```python
from build123d import *

# Parameters (mm, degrees)
F0_R     = 30
F1_DEPTH = 10
F2_R     = 2.5
F3_DEPTH = 10.001
F4_R     = 9
F5_DEPTH = 1.5
F6_R     = 7.5
F7_DEPTH = 10


with BuildPart() as f1:
    # F0 (on Top) → F1 (new body)
    with BuildSketch(Plane.XY):
        Circle(F0_R)
    extrude(amount=F1_DEPTH)

    # F2 (on face) → F3 (cut, through all)
    with BuildSketch(Plane.XY.offset(10)):
        with BuildLine():
            ThreePointArc((0, 23), (1.767767, 23.732233), (2.5, 25.5))
            ThreePointArc((2.5, 25.5), (-1.767767, 27.267767), (0, 23))
        make_face()
        with Locations((25.5, 0)):
            Circle(F2_R)
        with Locations((0, -25.5)):
            Circle(F2_R)
        with Locations((-25.5, 0)):
            Circle(F2_R)
    extrude(amount=-F3_DEPTH, mode=Mode.SUBTRACT)

    # F4 (on face) → F5 (join)
    with BuildSketch(Plane(origin=(0, 0, 0), x_dir=(1, 0, 0), z_dir=(0, 0, -1))):
        Circle(F4_R)
    extrude(amount=F5_DEPTH)

    # F6 (on face) → F7 (join)
    with BuildSketch(Plane(origin=(0, 0, -1.5), x_dir=(1, 0, 0), z_dir=(0, 0, -1))):
        Circle(F6_R)
    extrude(amount=F7_DEPTH)


solid = f1.part
```
Build history of the part. All positions in model axes, mm. A direction names the side the tool comes from. Round coordinates to 2 decimals unless told otherwise and drop trailing zeros. Order: outer loops, then holes, each group sorted by start corner. A loop starts at its lowest first (then second) coordinate and runs counter-clockwise, first axis right, second up. Notation, with made-up numbers: (36.5, 1) -> (51.5, 1) arc R24 cw to (51.5, 21) -> close; hole circle Ø3 at (-2, 5.25). An arc over 180 degrees is marked (long way). Answer in a Markdown table with one row per item.
1) Band-saw the part on A-A on y = 0. Give the cut face in (x, z).
Values:
| item | result |
|---|---|
| outline | (-30, 0) -> (-28, 0) -> (-28, 10) -> (-30, 10) -> close; (-23, 0) -> (-9, 0) -> (-9, -1.5) -> (-7.5, -1.5) -> (-7.5, -11.5) -> (7.5, -11.5) -> (7.5, -1.5) -> (9, -1.5) -> (9, 0) -> (23, 0) -> (23, 10) -> (-23, 10) -> close; (28, 0) -> (30, 0) -> (30, 10) -> (28, 10) -> close |
2) Which spindle directions (+Z, -Z, +X, -X, +Y, -Y) get a long thin tool onto all of the face, cutting with end or side? Do faces 4 (the cylindrical face through (-28, 0, 5)), 5 (the cylindrical face through (-1.172, -8.923, -0.74)). Say none if no direction does.
Values:
| item | result |
|---|---|
| face 4 | +Z, -Z |
| face 5 | -Z |
3) Band-saw the part on C-C on y = -25.5. Give the cut face in (x, z), and give its area (3 significant figures).
Values:
| item | result |
|---|---|
| outline | (-15.8, 0) -> (-2.5, 0) -> (-2.5, 10) -> (-15.8, 10) -> close; (2.5, 0) -> (15.8, 0) -> (15.8, 10) -> (2.5, 10) -> close |
| area | 266 mm2 |
4) Band-saw the part on B-B on z = 5.25. Give the cut face in (x, y), and give its area (3 significant figures).
Values:
| item | result |
|---|---|
| outline | circle Ø60 at (0, 0); hole circle Ø5 at (-25.5, 0); hole circle Ø5 at (0, -25.5); hole circle Ø5 at (0, 25.5); hole circle Ø5 at (25.5, 0) |
| area | 2,750 mm2 |
5) Mould opens along Y. For faces 1 (the cylindrical face through (-29.97, 1.32, 4.93)), 2 (the flat face through (0, 0, -11.5)), 3 (the cylindrical face through (0, -23, 5)) say: released by +Y, released by -Y, zero draft, split by the parting line, or undercut.
Values:
| item | result |
|---|---|
| face 1 | split by the parting line |
| face 2 | zero draft |
| face 3 | undercut |
6) Wall check: L1, parallel to Y at x = 0, z = 5; L2, parallel to Y at x = 1, z = 4.25; L3, parallel to X at y = -2, z = 1. Give the ranges that are in metal, low to high.
Values:
| item | result |
|---|---|
| L1 | -30 to -28, -23 to 23, 28 to 30 |
| L2 | -29.98 to -27.79, -23.21 to 23.21, 27.79 to 29.98 |
| L3 | -29.93 to -27, -24 to 24, 27 to 29.93 |
7) Pin check, flat tips, straight feed: P1, Ø4, axis at x = 6.5, y = -9, coming from the -Z side; P2, Ø12, axis at x = -22, z = 0.5, coming from the -Y side; P3, Ø10, axis at y = 22, z = 3.5, coming from the -X side; P4, Ø1, axis at x = -8.5, z = -8, coming from the +Y side. Stop position of each tip, or through.
Values:
| item | result |
|---|---|
| P1 | z = 0 |
| P2 | y = -25.38 |
| P3 | x = -24.72 |
| P4 | through |
